from build123d import *

# Parameters (mm, degrees)
F0_W     = 127
F0_H     = 127
F1_DEPTH = 63.5
F4_R     = 5


with BuildPart() as f1:
    # F0 (on Top) → F1 (new body, symmetric)
    with BuildSketch(Plane.XY):
        Rectangle(F0_W, F0_H)
    extrude(amount=F1_DEPTH, both=True)

    # F4
    f4_edges = [f1.edges().sort_by_distance(p)[0] for p in [
        (63.5, 0, 63.5),
        (0, 63.5, 63.5),
        (-63.5, 0, 63.5),
        (0, -63.5, 63.5),
        (0, -63.5, -63.5),
        (63.5, -63.5, 0),
        (-63.5, -63.5, 0),
        (63.5, 0, -63.5),
        (63.5, 63.5, 0),
        (0, 63.5, -63.5),
        (-63.5, 0, -63.5),
        (-63.5, 63.5, 0),
    ]]
    fillet(f4_edges, radius=F4_R)

    # F3 (on 3pt) → F5 (revolve)
    with BuildSketch(Plane(origin=(0, 0, 0), x_dir=(0.7071067812, 0.7071067812, 0), z_dir=(0.7071067812, -0.7071067812, 0))):
        Polygon((-106.1445555206, -75.0555349947), (106.1445555206, 75.0555349947), (104.412504713, 77.5050247374), (-107.8766063282, -72.6060452519), align=None)
    revolve(axis=Axis((0, 0, 0), (0.5773502692, 0.5773502692, 0.5773502692)))


solid = f1.part
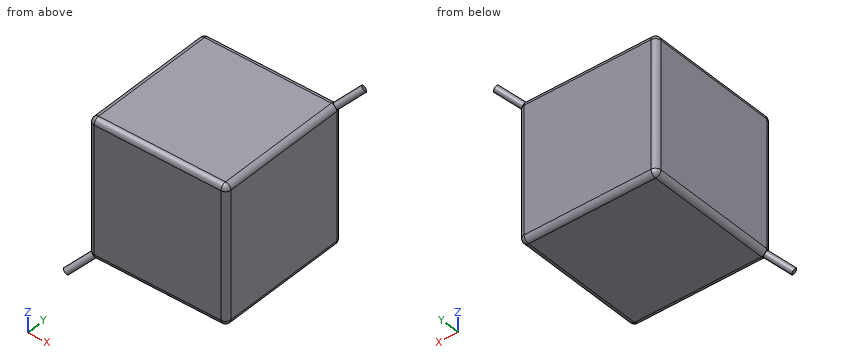
Here's how the part is built. I have some questions about the finished solid (model axes, mm). Coordinates: 2 decimals unless noted, no trailing zeros. Write each loop counter-clockwise with the first axis right and the second up, starting at its lowest first coordinate (ties: lowest second). Pieces come first, ordered by that corner, then holes.
Item 1: I want a section at A-A on z = 20. Write out the boundary of the cut face in (x, y).
Item 2: If I drill on line 1 (X direction, y = 42.5, z = -50.5), over which ranges is the centre line in solid material (lowest first)?
Item 3: Will these pins go through, and if not, where does the flat tip stop? pin 1 (6 mm diameter, centred on x = 2, y = 26.5, fed in from -Z); pin 2 (1.5 mm diameter, centred on x = 14.5, z = 49.5, fed in from -Y); pin 3 (1 mm diameter, centred on x = 41, z = 41, fed in from +Y).
Findings below:
1. outline: (-63.5, -58.5) arc R5 ccw to (-58.5, -63.5) - (58.5, -63.5) arc R5 ccw to (63.5, -58.5) - (63.5, 58.5) arc R5 ccw to (58.5, 63.5) - (-58.5, 63.5) arc R5 ccw to (-63.5, 58.5) - close
2. line 1: x = -63.5 to 63.5
3. pin 1: stops at z = -63.5
3. pin 2: stops at y = -63.5
3. pin 3: stops at y = 63.5
